Here's how the part is built. I have some questions about the finished solid (model axes, mm). Coordinates: 2 decimals unless noted, no trailing zeros. Loops run counter-clockwise (first coordinate to the right, second up) from the corner with the lowest first, then second, coordinate; pieces in that order, holes last. Notation, with made-up numbers: M 34,64 L 42,64 A26 cw 42,87 Z; hole C 34,-27 d10. An arc over 180 degrees is marked long. Use one line per item in the form item = value. Start each with the question number.
(1) Thinking about a two-plate mould opening in Y: for faces 1 (the cylindrical face through (33.44, -19.72, 4.92)), 2 (the cylindrical face through (0.36, 38.82, 3.51)), 3 (the flat face through (-9, 8, 0)), which applies, +Y half, -Y half, draft (parallel to the pull), parting line (faces both ways), or undercut?
(2) Imagine slicing it at B-B, the plane y = 8.5. Please give me the cut outline in (x, z).
(3) Will these pins go through, and if not, where does the flat tip stop? P1, Ø4, axis at x = 28.5, z = 1, coming from the -Y side; P2, Ø4, axis at y = 13, z = 2, coming from the +X side; P3, Ø20, axis at x = 0, y = 0, coming from the -Z side; P4, Ø2, axis at y = -8, z = 1.5, coming from the -X side.
(4) Please list where these lines run through material, in increasing order: L1, parallel to Y at x = 0, z = 5; L2, parallel to Y at x = -3.5, z = 6.25; L3, parallel to X at y = -7, z = 5.
(5) Imagine slicing it at D-D, the plane y = -17.5. State how many separate pieces and enclosed holes the cut face has, and give its area (3 significant figures).
(6) Imagine slicing it at A-A, the plane x = 0. Please give me the cut outline in (y, z).
(7) Imagine slicing it at C-C, the plane z = 1.5. Please give me the cut outline in (x, y), and give its area (3 significant figures).
```python
from build123d import *
from build123d import SkipClean  # not in build123d's __all__

# Parameters (mm, degrees)
F0_R         = 11.0744
F1_DEPTH     = 7.112
F3_T3_ANGLE  = 270.1069651298
F3_S4_R      = 24.9492229885
F3_T5_DEPTH  = 22
F3_T8_ANGLE  = 270.1069651298
F3_S9_R      = 24.9492229885
F3_T10_DEPTH = 22


# Not quite as in the source:
# - a fillet or chamfer that OpenCascade refuses, or shapes differently, is made with other operations: its cross-section is extruded or revolved along the edge and cut away or added
# - a feature of the source that left no trace in its solid (it failed there, or was rolled back) is left out
# - a pattern or mirror of a feature is missing from the dataset's text; its kind, count and spacing are read off the source's solid


with BuildPart() as f1:
    # F0 (on Top) → F1 (new body)
    with BuildSketch(Plane.XY):
        with BuildLine():
            ThreePointArc((-10.7982111441, 22.491384213), (-1.236653926, 35.9543591725), (11.0744, 24.9492229885))
            ThreePointArc((11.0744, 24.9492229885), (11.005136184, 23.7125690625), (10.7982111441, 22.491384213))
            ThreePointArc((10.7982111441, 22.491384213), (12.0832280354, 21.8279483226), (13.3276464943, 21.0911727187))
            ThreePointArc((13.3276464943, 21.0911727187), (0, 38.824045977), (-13.3276464943, 21.0911727187))
            ThreePointArc((-13.3276464943, 21.0911727187), (-12.0832280354, 21.8279483226), (-10.7982111441, 22.491384213))
        make_face()
        with BuildLine():
            ThreePointArc((10.7982111441, 22.491384213), (0, 13.8748229885), (-10.7982111441, 22.491384213))
            ThreePointArc((-10.7982111441, 22.491384213), (-12.0832280354, 21.8279483226), (-13.3276464943, 21.0911727187))
            ThreePointArc((-13.3276464943, 21.0911727187), (-12.7649941961, 19.5117938041), (-12.0159491811, 18.0118114943))
            ThreePointArc((-12.0159491811, 18.0118114943), (-12.0159491811, 6.9374114943), (-21.6066609127, 1.4002114943))
            ThreePointArc((-21.6066609127, 1.4002114943), (-23.2802062059, 1.2989123509), (-24.9293146172, 0.9964940774))
            ThreePointArc((-24.9293146172, 0.9964940774), (-24.9451717776, -0.4495917229), (-24.8772156668, -1.8941669402))
            ThreePointArc((-24.8772156668, -1.8941669402), (-15.0331191052, -3.5622109498), (-10.5322609127, -12.4746114943))
            ThreePointArc((-10.5322609127, -12.4746114943), (-11.4576064423, -16.9062058706), (-14.0790045227, -20.5972172728))
            ThreePointArc((-14.0790045227, -20.5972172728), (-12.8619437422, -21.3783565997), (-11.6016681229, -22.0876667961))
            ThreePointArc((-11.6016681229, -22.0876667961), (-10.5152120097, -20.8107061551), (-9.5907117317, -19.4120229885))
            ThreePointArc((-9.5907117317, -19.4120229885), (0, -13.8748229885), (9.5907117317, -19.4120229885))
            ThreePointArc((9.5907117317, -19.4120229885), (10.5152120097, -20.8107061551), (11.6016681229, -22.0876667961))
            ThreePointArc((11.6016681229, -22.0876667961), (12.8619437422, -21.3783565997), (14.0790045227, -20.5972172728))
            ThreePointArc((14.0790045227, -20.5972172728), (12.0159491811, -6.9374114943), (24.8772156668, -1.8941669402))
            ThreePointArc((24.8772156668, -1.8941669402), (24.9312146589, -0.947767568), (24.9492229885, 0))
            ThreePointArc((24.9492229885, 0), (24.9442453991, 0.4983464632), (24.9293146172, 0.9964940774))
            ThreePointArc((24.9293146172, 0.9964940774), (23.2802062059, 1.2989123509), (21.6066609127, 1.4002114943))
            ThreePointArc((21.6066609127, 1.4002114943), (12.0159491811, 6.9374114943), (12.0159491811, 18.0118114943))
            ThreePointArc((12.0159491811, 18.0118114943), (12.7649941961, 19.5117938041), (13.3276464943, 21.0911727187))
            ThreePointArc((13.3276464943, 21.0911727187), (12.0832280354, 21.8279483226), (10.7982111441, 22.491384213))
        make_face()
        Circle(F0_R, mode=Mode.SUBTRACT)
        with BuildLine():
            ThreePointArc((-12.0159491811, 18.0118114943), (-12.7649941961, 19.5117938041), (-13.3276464943, 21.0911727187))
            ThreePointArc((-13.3276464943, 21.0911727187), (-21.6066609127, 12.4746114943), (-24.9293146172, 0.9964940774))
            ThreePointArc((-24.9293146172, 0.9964940774), (-23.2802062059, 1.2989123509), (-21.6066609127, 1.4002114943))
            ThreePointArc((-21.6066609127, 1.4002114943), (-12.0159491811, 6.9374114943), (-12.0159491811, 18.0118114943))
        make_face()
        with BuildLine():
            ThreePointArc((24.9293146172, 0.9964940774), (21.6066609127, 12.4746114943), (13.3276464943, 21.0911727187))
            ThreePointArc((13.3276464943, 21.0911727187), (12.7649941961, 19.5117938041), (12.0159491811, 18.0118114943))
            ThreePointArc((12.0159491811, 18.0118114943), (12.0159491811, 6.9374114943), (21.6066609127, 1.4002114943))
            ThreePointArc((21.6066609127, 1.4002114943), (23.2802062059, 1.2989123509), (24.9293146172, 0.9964940774))
        make_face()
        with BuildLine():
            ThreePointArc((11.6016681229, -22.0876667961), (33.6226100938, -19.4120229885), (24.9293146172, 0.9964940774))
            ThreePointArc((24.9293146172, 0.9964940774), (24.9442453991, 0.4983464632), (24.9492229885, 0))
            ThreePointArc((24.9492229885, 0), (24.9312146589, -0.947767568), (24.8772156668, -1.8941669402))
            ThreePointArc((24.8772156668, -1.8941669402), (30.5190614572, -5.9010696867), (32.6810609127, -12.4746114943))
            ThreePointArc((32.6810609127, -12.4746114943), (26.0382552891, -22.6236659647), (14.0790045227, -20.5972172728))
            ThreePointArc((14.0790045227, -20.5972172728), (12.8619437422, -21.3783565997), (11.6016681229, -22.0876667961))
        make_face()
        with BuildLine():
            ThreePointArc((-9.5907117317, -19.4120229885), (-10.5152120097, -20.8107061551), (-11.6016681229, -22.0876667961))
            ThreePointArc((-11.6016681229, -22.0876667961), (0, -24.9492229885), (11.6016681229, -22.0876667961))
            ThreePointArc((11.6016681229, -22.0876667961), (10.5152120097, -20.8107061551), (9.5907117317, -19.4120229885))
            ThreePointArc((9.5907117317, -19.4120229885), (0, -13.8748229885), (-9.5907117317, -19.4120229885))
        make_face()
    extrude(amount=F1_DEPTH)

    # F1_copies: F1 across plane


with BuildPart() as f1_1:
    add(f1.part, clean=False)
    with SkipClean():  # cleaning this boolean's faces spoils the solid; the shape is the same uncleaned
        add(f1.part.mirror(Plane(origin=(0, 0, 0), x_dir=(-0.8660254038, 0.5, 0), z_dir=(-0.5, -0.8660254038, 0))), clean=False)

    # F3: fillet of radius 2.794 on 2 edges, made by hand


with BuildPart() as f3_tool1:
    # F3_s2 → F3_t3 (revolve)
    with BuildSketch(Plane(origin=(4.5458669208, -17.0289729971, 0), x_dir=(0, 0, 1), z_dir=(-0.2579172921, 0.9661669993, 0))):
        with BuildLine():
            ThreePointArc((0, 6.5774017335), (0.8183436534, 4.6017453869), (2.794, 3.7834017335))
            Line((2.794, 3.7834017335), (0, 3.7834017335))
            Line((0, 3.7834017335), (0, 6.5774017335))
        make_face()
    revolve(axis=Axis((21.6066609127, -12.4746114943, 0), (0, 0, 1)), revolution_arc=F3_T3_ANGLE)

    # F3_s4 → F3_t5 (cut, symmetric)
    with BuildSketch(Plane.XY.offset(2.4)):
        Circle(F3_S4_R)
    extrude(amount=F3_T5_DEPTH, both=True, mode=Mode.SUBTRACT)


with BuildPart() as f3_tool6:
    # F3_s7 → F3_t8 (revolve)
    with BuildSketch(Plane(origin=(-4.5458669208, -17.0289729971, 0), x_dir=(0, 0, 1), z_dir=(0.2579172921, 0.9661669993, 0))):
        with BuildLine():
            ThreePointArc((7.112, -6.5774017335), (6.2936563466, -4.6017453869), (4.318, -3.7834017335))
            Line((4.318, -3.7834017335), (7.112, -3.7834017335))
            Line((7.112, -3.7834017335), (7.112, -6.5774017335))
        make_face()
    revolve(axis=Axis((-21.6066609127, -12.4746114943, 7.112), (0, 0, -1)), revolution_arc=F3_T8_ANGLE)

    # F3_s9 → F3_t10 (cut, symmetric)
    with BuildSketch(Plane.XY.offset(5.7)):
        Circle(F3_S9_R)
    extrude(amount=F3_T10_DEPTH, both=True, mode=Mode.SUBTRACT)


with BuildPart() as f1_2:
    add(f1_1.part, clean=False)

    # F3_t11: cut F3_tool1, F3_tool6
    add([f3_tool1.part, f3_tool6.part], mode=Mode.SUBTRACT)


solid = f1_2.part
```
Answer:
q1.face_1 = parting line
q1.face_2 = undercut
q1.face_3 = draft
q2.outline = M -23.46,0 L -7.1,0 L -7.1,7.11 L -23.46,7.11 Z; M 7.1,0 L 23.46,0 L 23.46,7.11 L 7.1,7.11 Z
q3.P1 = -25.23
q3.P2 = 22.39
q3.P3 = through
q3.P4 = -35.04
q4.L1 = -24.95 to -11.07, 11.07 to 13.87, 36.02 to 38.82
q4.L2 = -24.7 to -10.51, 10.51 to 14.44, 35.46 to 38.38
q4.L3 = -34.26 to -31.23, -11.98 to -8.58, 8.58 to 11.98, 31.23 to 34.36
q5.separate_pieces = 3
q5.enclosed_holes = 0
q5.area = 207 mm²
q6.outline = M -24.95,0 L -11.07,0 L -11.07,7.11 L -24.95,7.11 Z; M 11.07,0 L 13.87,0 L 13.87,7.11 L 11.07,7.11 Z; M 36.02,0 L 38.82,0 L 38.82,7.11 L 36.02,7.11 Z
q7.outline = M -24.93,1 A13.87 ccw long -11.6,-22.09 A24.95 ccw 11.89,-21.93 A13.56 ccw long 24.94,0.67 A24.95 ccw 13.33,21.09 A13.87 ccw long -13.33,21.09 A24.95 ccw Z; hole C -21.61,-12.47 d22.15; hole C 0,0 d22.15; hole C 0,24.95 d22.15; hole C 21.61,-12.47 d22.15
q7.area = 1,410 mm²
